Input: part model. Units: mm. Frame: model coordinates. Coordinates: 2 decimals unless noted, no trailing zeros. Loops run counter-clockwise (first coordinate to the right, second up) from the corner with the lowest first, then second, coordinate; pieces in that order, holes last. Notation, with made-up numbers: (23, 89.5) - (78, 89.5) arc R32 cw to (78, 116.5) - close; hole circle Ø6 at (-0.75, 8.25). An arc over 180 degrees is marked (long way). Use a Markdown table: item, result. Add a question column.
1. Contact query for flat-ended pins moving along their axis: P1, Ø5, axis at x = 0, y = 157.5, coming from the +Z side; P2, Ø3, axis at y = 21, z = -5.5, coming from the +X side; P3, Ø5.5, axis at x = 3.5, y = 67, coming from the -Z side; P4, Ø2, axis at y = 159, z = -4, coming from the -X side. Output: stop coordinate, or through.
2. Section query A-A on y = 131.5. Return the cut outline in (x, z).
3. Section query B-B on y = 19. Return the cut outline in (x, z), then the cut area to 3 significant figures.
4. Ray query, L1, parallel to Z at x = 8.25, y = 42; L2, parallel to Y at x = 7, z = -3; L3, parallel to Z at x = 6.75, y = 53. Return the intervals inside material, ascending. Write a range as [from, to].
Autodesk Inventor part; units mm, degrees
ref_plane "YZ Plane" through (0, 0, 0) normal (1, 0, 0) x (0, 1, 0)
ref_plane "XZ Plane" through (0, 0, 0) normal (0, 1, 0) x (-1, 0, 0)
ref_plane "XY Plane" through (0, 0, 0) normal (0, 0, 1) x (1, 0, 0)
sketch "草圖1" plane through (0, 0, 0) normal (0, 1, 0) x (-1, 0, 0)
  line L0 (0, 0) -> (-10, 0)
  line L1 (-10, 0) -> (-10, -10)
  line L2 (-10, -10) -> (0, -10)
  line L3 (0, -10) -> (0, 0)
  dimension "d0" = 10
  dimension "d1" = 10
extrude "擠出1" add sketch "草圖1" along normal blind 50
chamfer "倒角1" distance 2.4 angle 45 4 edges at (5, 50, 0) (10, 50, -5) (5, 50, -10) (0, 50, -5)
sketch "草圖2" plane through (0, 50, 0) normal (0, 1, 0) x (1, 0, 0)
  line L0 (2.4, 2.4) -> (2.4, 7.6)
  line L1 (7.6, 2.4) -> (2.4, 2.4)
  line L2 (2.4, 7.6) -> (7.6, 7.6)
  line L3 (7.6, 7.6) -> (7.6, 2.4)
  line L4 (7.6, 2.4) -> (2.4, 2.4)
  line L5 (2.4, 2.4) -> (2.4, 7.6)
  point P0 (0, 0)
extrude "擠出2" add sketch "草圖2" along normal blind 30
sketch "草圖3" plane through (0, 80, 0) normal (0, 1, 0) x (1, 0, 0)
  line L0 (2.4, 7.6) -> (7.6, 7.6)
  line L1 (7.6, 7.6) -> (7.6, 2.4)
  line L2 (7.6, 2.4) -> (2.4, 2.4)
  line L3 (2.4, 2.4) -> (2.4, 7.6)
  circle A0 centre (5, 5) radius 7.0711
  line L4 (7, 7) -> (3, 7)
  line L5 (3, 7) -> (3, 3)
  line L6 (3, 3) -> (7, 3)
  line L7 (7, 3) -> (7, 7)
  line L8 (7, 7) -> (3, 3) construction
  line L9 (3, 7) -> (7, 3) construction
  point P0 (0, 0)
  point P1 (10, 10)
  dimension "d31" = 4
  dimension "d32" = 4
extrude "擠出3" add sketch "草圖3" along normal blind 110 contours L7 L6 L5 L4
extrude "擠出5" add sketch "草圖3" along normal blind 1 contours A0
fillet "圓角1" radius 0.2 2 edges at (-2.0711, 80, -5) (-2.0711, 81, -5)
chamfer "倒角7" distance 1.25 angle 45 4 edges at (5, 190, -7) (7, 190, -5) (5, 190, -3) (3, 190, -5)
extrude "擠出6" add sketch "草圖3" along normal blind 2 contours L0 L1 L2 L3 | L7 L6 L5 L4
chamfer "倒角8" distance 1 angle 30 1 edges at (5, 82, -7.6) measured on face at (5.8667, 81.3333, -7.6)
chamfer "倒角9" distance 1 angle 30 1 edges at (2.4, 82, -4.7116) measured on face at (2.4, 81.3333, -5.6744)
chamfer "倒角10" distance 1 angle 30 1 edges at (5.2884, 82, -2.4) measured on face at (4.3256, 81.3333, -2.4)
chamfer "倒角11" distance 1 angle 30 1 edges at (7.6, 82, -5) measured on face at (7.6, 81.3333, -5.6744)
sketch "草圖7" plane through (0, 190, 0) normal (0, 1, 0) x (1, 0, 0)
  line L0 (5.75, 5.75) -> (5.75, 4.25)
  circle A0 centre (5, 5) radius 0.725
  line L1 (5.75, 5) -> (4.25, 5)
  point P0 (0, 0)
  point P1 (5.725, 5)
  point P2 (4.275, 5)
  dimension "d54" = 1.45
revolve "迴轉2" add sketch "草圖7" angle 180 about axis through (5.75, 190, -5) along (-1, 0, 0) picked at (4.7654, 4.9422) contours A0 L1
sketch "草圖9" plane through (0, 190, 0) normal (0, 1, 0) x (1, 0, 0)
  circle A0 centre (5, 5) radius 0.725
  circle A1 centre (5, 5) radius 0.75
  point P0 (0, 0)
extrude "擠出8" add sketch "草圖9" along normal blind 0.1 contours A0 | A1
properties part number "尖尖"
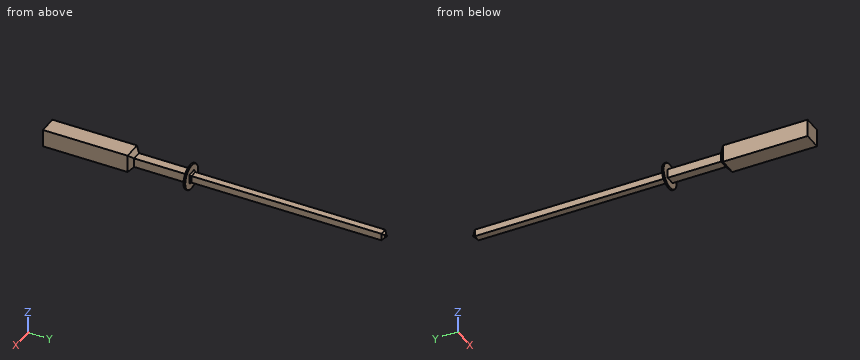
Resolved:
| question | item | result |
|---|---|---|
| 1 | P1 | through |
| 1 | P2 | x = 10 |
| 1 | P3 | z = -7.6 |
| 1 | P4 | x = 3 |
| 2 | outline | (3, -7) - (7, -7) - (7, -3) - (3, -3) - close |
| 3 | outline | (0, -10) - (10, -10) - (10, 0) - (0, 0) - close |
| 3 | area | 100 mm² |
| 4 | L1 | [-10, 0] |
| 4 | L2 | [0, 82] |
| 4 | L3 | [-7.6, -2.4] |
